Autodesk Inventor part; units mm, degrees
ref_plane "YZ Plane" through (0, 0, 0) normal (1, 0, 0) x (0, 1, 0)
ref_plane "XZ Plane" through (0, 0, 0) normal (0, 1, 0) x (-1, 0, 0)
ref_plane "XY Plane" through (0, 0, 0) normal (0, 0, 1) x (1, 0, 0)
sketch "Sketch1" plane through (0, 0, 0) normal (0, 1, 0) x (-1, 0, 0)
  line L0 (63.5, 88.9) -> (-63.5, 88.9)
  line L1 (-63.5, 88.9) -> (-63.5, -88.9)
  line L2 (-63.5, -88.9) -> (63.5, -88.9)
  line L3 (63.5, -88.9) -> (63.5, 88.9)
  line L4 (63.5, 88.9) -> (-63.5, -88.9) construction
  line L5 (-63.5, 88.9) -> (63.5, -88.9) construction
  point P0 (0, 0)
  dimension "d0" = 127
  dimension "d1" = 177.8
extrude "Extrusion1" add sketch "Sketch1" along normal blind 12.7
sketch "Sketch2" plane through (0, 12.7, 0) normal (0, 1, 0) x (1, 0, 0)
  circle A0 centre (0, 25.4) radius 51.0159
  line L0 (-63.5, 88.9) -> (-63.5, -88.9)
  line L1 (63.5, 88.9) -> (-63.5, 88.9)
  point P0 (0, 0)
  dimension "d4" = 102.0318
  dimension "d5" = 63.5
  dimension "d6" = 63.5
sketch "Sketch3" plane through (0, 12.7, 0) normal (0, 1, 0) x (1, 0, 0)
  arc A0 (-24.2412, -32.7116) -> (24.2412, -32.7116) centre (0, -47.8409) ccw
  line L0 (-24.2412, -32.7116) -> (-17.8095, -22.4063)
  line L1 (0, 124.46) -> (0, -124.46)
  line L2 (24.2412, -32.7116) -> (17.8095, -22.4063)
  arc A1 (17.8095, -22.4063) -> (-17.8095, -22.4063) centre (0, -33.5215) ccw
  circle A2 centre (0, -47.8409) radius 22.225 construction
  circle A3 centre (0, 25.4) radius 51.0159
  point P0 (0, 0)
  dimension "d13" = 57.15
  dimension "d14" = 70
  dimension "d58" = 44.45
extrude "Extrusion3" cut sketch "Sketch3" against normal through all contours L0 A3 L1 A0 | L1 A3 L2 A0 | A1 L1 A3 | L1 A1 A3 picked at (-3.4245, -21.2764) picked at (3.4245, -21.2764)
sketch "Sketch5" plane through (0, 12.7, 0) normal (0, 1, 0) x (1, 0, 0)
  line L0 (-34.925, -35.1409) -> (-30.2521, -26.8409)
  line L1 (-30.2521, -26.8409) -> (-27.4855, -28.3985)
  line L2 (-27.4855, -28.3985) -> (-31.75, -35.9732)
  line L3 (-31.75, -35.9732) -> (-31.75, -59.7086)
  line L4 (-31.75, -59.7086) -> (-27.4855, -67.2833)
  line L5 (-27.4855, -67.2833) -> (-30.2521, -68.8409)
  line L6 (-34.925, -35.1409) -> (-34.925, -60.5409)
  line L7 (-34.925, -60.5409) -> (-30.2521, -68.8409)
  arc A0 (-24.2412, -32.7116) -> (24.2412, -32.7116) centre (0, -47.8409) ccw
  arc A1 (-24.2412, -32.7116) -> (24.2412, -32.7116) centre (0, -47.8409) ccw construction
  line L8 (-28.575, -47.8409) -> (28.575, -47.8409) construction
  line L9 (0, 124.46) -> (0, -124.46) construction
  line L10 (34.925, -35.1409) -> (30.2521, -26.8409)
  line L11 (30.2521, -26.8409) -> (27.4855, -28.3985)
  line L12 (27.4855, -28.3985) -> (31.75, -35.9732)
  line L13 (31.75, -35.9732) -> (31.75, -59.7086)
  line L14 (31.75, -59.7086) -> (27.4855, -67.2833)
  line L15 (27.4855, -67.2833) -> (30.2521, -68.8409)
  line L16 (34.925, -35.1409) -> (34.925, -60.5409)
  line L17 (34.925, -60.5409) -> (30.2521, -68.8409)
  point P0 (0, 0)
  point P1 (-31.75, -47.8409)
  point P2 (31.75, -47.8409)
  dimension "d16" = 3.175
  dimension "d17" = 3.175
  dimension "d18" = 3.175
  dimension "d19" = 42
  dimension "d20" = 25.4
  dimension "d21" = 9.525
  dimension "d22" = 63.5
extrude "Extrusion4" add sketch "Sketch5" along normal blind 25.4
sketch "Sketch6" plane through (0, 38.1, 0) normal (0, 1, 0) x (1, 0, 0)
  line L0 (-30.2521, -68.8409) -> (-27.4855, -67.2833)
  line L1 (27.4855, -67.2833) -> (30.2521, -68.8409)
  line L2 (31.75, -59.7086) -> (27.4855, -67.2833)
  line L3 (31.75, -35.9732) -> (31.75, -59.7086)
  line L4 (27.4855, -28.3985) -> (31.75, -35.9732)
  line L5 (30.2521, -26.8409) -> (27.4855, -28.3985)
  line L6 (-27.4855, -28.3985) -> (-30.2521, -26.8409)
  line L7 (-31.75, -35.9732) -> (-27.4855, -28.3985)
  line L8 (-31.75, -59.7086) -> (-31.75, -35.9732)
  line L9 (-27.4855, -67.2833) -> (-31.75, -59.7086)
  line L10 (-30.2521, -68.8409) -> (30.2521, -68.8409)
  line L11 (30.2521, -26.8409) -> (-30.2521, -26.8409)
  point P0 (0, 0)
extrude "Extrusion5" add sketch "Sketch6" against normal blind 3.175
sketch "Sketch7" plane through (0, 38.1, 0) normal (0, 1, 0) x (1, 0, 0)
  arc A0 (-24.2412, -32.7116) -> (24.2412, -32.7116) centre (0, -47.8409) ccw
  line L0 (21, -68.8409) -> (-21, -68.8409) construction
  line L1 (-21, -68.8409) -> (-21, -26.8409) construction
  line L2 (-21, -26.8409) -> (21, -26.8409) construction
  line L3 (21, -26.8409) -> (21, -68.8409) construction
  line L4 (21, -68.8409) -> (-21, -26.8409) construction
  line L5 (-21, -68.8409) -> (21, -26.8409) construction
  line L6 (15.5, -63.3409) -> (-15.5, -63.3409) construction
  line L7 (-15.5, -63.3409) -> (-15.5, -32.3409) construction
  line L8 (-15.5, -32.3409) -> (15.5, -32.3409) construction
  line L9 (15.5, -32.3409) -> (15.5, -63.3409) construction
  line L10 (15.5, -63.3409) -> (-15.5, -32.3409) construction
  line L11 (-15.5, -63.3409) -> (15.5, -32.3409) construction
  circle A1 centre (0, -47.8409) radius 12.7
  point P0 (0, 0)
  dimension "d27" = 42
  dimension "d28" = 42
  dimension "d29" = 31
  dimension "d30" = 31
  dimension "d31" = 25.4
extrude "Extrusion6" cut sketch "Sketch7" against normal through all
hole "Hole1" at (-15.5, 38.1, 63.3409) at (15.5, 38.1, 63.3409) at (15.5, 38.1, 32.3409) at (-15.5, 38.1, 32.3409) direction (0, -1, 0) diameter 2.5 depth 3.175 tip angle 118
sketch "Sketch8" plane through (0, 12.7, 0) normal (0, 1, 0) x (1, 0, 0)
  line L0 (-53.975, -12.7) -> (-50.8, -12.7)
  line L1 (-50.8, -12.7) -> (-50.8, 0)
  line L2 (-50.8, 0) -> (-53.975, 0)
  line L3 (-53.975, 0) -> (-53.975, -12.7)
  line L4 (-51.0159, 25.4) -> (51.0159, 25.4) construction
  line L5 (0, -25.6159) -> (0, 76.4159) construction
  point P0 (0, 0)
  point P1 (0, 25.4)
  point P2 (0, 25.4)
  dimension "d41" = 12.7
  dimension "d42" = 3.175
  dimension "d43" = 25.4
  dimension "d44" = 50.8
extrude "Extrusion7" add sketch "Sketch8" along normal blind 13.462
sketch "Sketch9" plane through (-53.975, 12.7, 0) normal (-1, 0, 0) x (0, 0, 1)
  line L0 (12.7, 13.462) -> (0, 13.462)
  arc A0 (12.7, 13.462) -> (0, 13.462) centre (6.35, 13.462) ccw
  point P0 (0, -12.7)
extrude "Extrusion8" add sketch "Sketch9" against normal blind 3.175
hole "Hole2" at (-53.975, 26.162, 6.35) direction (1, 0, 0) diameter 6.731 depth 3.175 tip angle 118
ref_plane "Work Plane1" through (-51.0159, 12.7, -25.4) normal (0, 0, 1) x (1, 0, 0)
ref_plane "Work Plane2" through (0, 12.7, 25.6159) normal (1, 0, 0) x (0, 0, -1)
mirror "Mirror1" about plane through (-51.0159, 12.7, -25.4) normal (0, 0, 1) of "Extrusion7", "Extrusion8", "Hole2"
mirror "Mirror2" about plane through (0, 12.7, 25.6159) normal (1, 0, 0) of "Extrusion7", "Extrusion8", "Hole2", "Mirror1"
sketch "Sketch11" plane through (0, 12.7, 0) normal (0, 1, 0) x (1, 0, 0)
  circle A0 centre (0, 25.4) radius 51.0159
  circle A1 centre (0, 25.4) radius 9.0805
  circle A2 centre (0, 25.4) radius 5.9055
  point P0 (0, 0)
  dimension "d59" = 18.161
  dimension "d60" = 3.175
extrude "Extrusion9" add sketch "Sketch11" along normal blind 9.525 contours A1
equation "\"d0\" = base_width"
equation "\"d1\" = base_length"
equation "\"d2\" = base_height"
equation "\"d6\" = d5"
equation "\"d14\" = base_cutout_contact_angle"
equation "\"d58\" = base_cutout_diameter"
equation "\"d16\" = turntable_motor_support_thickness"
equation "\"d17\" = turntable_motor_support_thickness"
equation "\"d18\" = turntable_motor_support_thickness"
equation "\"d22\" = turntable_motor_support_width"
equation "\"d23\" = turntable_motor_support_height"
equation "\"d25\" = turntable_motor_support_thickness"
equation "\"d31\" = turntable_motor_boss"
equation "\"d32\" = turntable_motor_support_thickness"
equation "\"d39\" = turntable_motor_support_thickness"
equation "\"d54\" = turntable_motor_support_thickness"
equation "\"d61\" = turntable_ring_height"
equation "\"base_length\" = 177.8"
equation "\"base_width\" = 127"
equation "\"base_height\" = 12.7"
equation "\"turntable_diameter\" = 101.6"
equation "\"turntable_height\" = 9.525"
equation "\"turntable_spur_width\" = 6.35"
equation "\"spine_diameter\" = 31.75"
equation "\"spine_height\" = 25.4"
equation "\"shoulder_length\" = 50.8"
equation "\"shoulder_width\" = 69.85"
equation "\"shoulder_wall_thickness\" = 4.7625"
equation "\"shoulder_gear_diameter\" = 63.5"
equation "\"shoulder_motor_gear_diameter\" = 25.4"
equation "\"shoulder_gear_shaft_diameter\" = 12.7"
equation "\"shoulder_motor_boss\" = 25.4"
equation "\"turntable_bed_depth\" = 0"
equation "\"base_cutout_diameter\" = 44.45"
equation "\"base_turntable_contact_angle\" = 60deg"
equation "\"base_cutout_contact_angle\" = 70deg"
equation "\"turntable_motor_support_thickness\" = 3.175"
equation "\"turntable_motor_support_height\" = 25.4"
equation "\"turntable_motor_boss\" = 25.4"
equation "\"turntable_motor_support_width\" = 63.5"
equation "\"turntable_retention_shaft_diameter\" = 6.35"
equation "\"turntable_retention_shaft_length\" = 152.4"
equation "\"shoulder_gear_thickness\" = 6.35"
equation "\"arm_distal_length\" = 152.4"
equation "\"arm_proximal_length\" = 203.2"
equation "\"arm_proximal_central_diameter\" = 25.4"
equation "\"arm_proximal_thickness\" = 9.525"
equation "\"arm_proximal_motor_boss\" = 25.4"
equation "\"turntable_ring_height\" = 9.525"
equation "\"turntable_ring_diameter\" = 19.05"
properties part number "base"
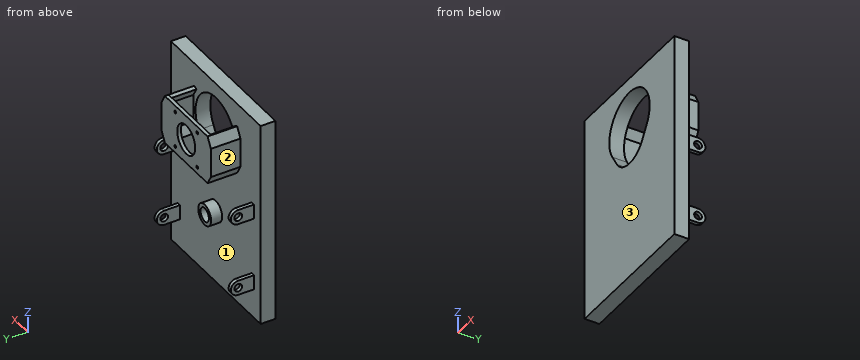
Verification items for the finished model (mm, model axes). Face numbers are marked on the shaded views. Coordinates: 2 decimals unless noted, no trailing zeros. Order: outer loops, then holes, each group sorted by start corner. A loop starts at its lowest first (then second) coordinate and runs counter-clockwise, first axis right, second up. Notation, with made-up numbers: M -5.5,21.5 L 52.5,21.5 A29 ccw 52.5,41.5 Z; hole C -32,-13 d1. An arc over 180 degrees is marked long. Return JSON: item names as keys, results as strings.
1) Cross-section at B-B, the plane x = 0. Record the boundary of the cut face in (y, z) (1 decimal).
Answer list:
{"outline": "M 0,-88.9 L 12.7,-88.9 L 12.7,-34.5 L 22.2,-34.5 L 22.2,-31.3 L 12.7,-31.3 L 12.7,-19.5 L 22.2,-19.5 L 22.2,-16.3 L 12.7,-16.3 L 12.7,12.5 L 0,12.5 Z; M 0,76.4 L 12.7,76.4 L 12.7,88.9 L 0,88.9 Z; M 34.9,26.8 L 38.1,26.8 L 38.1,35.1 L 34.9,35.1 Z; M 34.9,60.5 L 38.1,60.5 L 38.1,68.8 L 34.9,68.8 Z"}
2) Cross-section at A-A, the plane y = 20. Count the separate pieces of the cut face and the enclosed holes in it, and give its area (3 significant figures).
Answer list:
{"separate pieces": "7", "enclosed holes": "1", "area": "582 mm2"}
3) Thickness scan on L1, parallel to Z at x = 15.5, y = 35.9; L2, parallel to Y at x = -52.6, z = 6.35; L3, parallel to X at y = 17, z = -25. Record the ranges inside material, lowest first. Write a range as [from, to].
Answer list:
{"L1": "[26.84, 31.09], [33.59, 62.09], [64.59, 68.84]", "L2": "[0, 22.8], [29.53, 32.51]", "L3": "[-9.07, -5.89], [5.89, 9.07]"}
4) Gauge pin test, flat ends, axial feed: pin 1 (6.5 mm diameter, centred on y = 17.5, z = -60, fed in from -X) (3 decimals); pin 2 (8 mm diameter, centred on x = -26, y = 19.5, fed in from -Z); pin 3 (2.5 mm diameter, centred on x = 52, y = 19.5, fed in from +Z). Record the tip position at first contact, or that the pin passes through.
Answer list:
{"pin 1": "x = -53.975", "pin 2": "z = 26.98", "pin 3": "z = 12.7"}
5) Cross-section at D-D, the plane y = 7. Record the boundary of the cut face in (x, z), and give its area (3 significant figures).
Answer list:
{"outline": "M -63.5,-88.9 L 63.5,-88.9 L 63.5,88.9 L -63.5,88.9 Z; hole M -24.24,32.71 L -17.81,22.41 A20.99 ccw 17.81,22.41 L 24.24,32.71 A28.58 ccw long Z", "area": "19,800 mm2"}
6) Release check for a two-part mould opening along X. For the marked faces 1, 2 and 3 record: +X half, -X half, draft (parallel to the pull), parting line (faces both ways), or undercut.
Answer list:
{"face 1": "undercut", "face 2": "-X half", "face 3": "draft"}
7) Cross-section at C-C, the plane z = -57.15. Record the boundary of the cut face in (x, y) (1 decimal).
Answer list:
{"outline": "M -63.5,0 L 63.5,0 L 63.5,12.7 L 54,12.7 L 54,22.8 L 50.8,22.8 L 50.8,12.7 L -50.8,12.7 L -50.8,22.8 L -54,22.8 L -54,12.7 L -63.5,12.7 Z; M -54,29.5 L -50.8,29.5 L -50.8,32.5 L -54,32.5 Z; M 50.8,29.5 L 54,29.5 L 54,32.5 L 50.8,32.5 Z"}
